Autodesk Inventor part; units mm, degrees
ref_plane "YZ Plane" through (0, 0, 0) normal (1, 0, 0) x (0, 1, 0)
ref_plane "XZ Plane" through (0, 0, 0) normal (0, 1, 0) x (-1, 0, 0)
ref_plane "XY Plane" through (0, 0, 0) normal (0, 0, 1) x (1, 0, 0)
sketch "Sketch1" plane through (0, 0, 0) normal (0, 1, 0) x (-1, 0, 0)
  line L0 (0, 25.4) -> (25.4, 25.4)
  line L1 (25.4, 25.4) -> (25.4, 0)
  line L2 (25.4, 0) -> (0, 0)
  line L3 (0, 0) -> (0, 25.4)
  line L4 (22.225, 22.225) -> (3.175, 22.225)
  line L5 (3.175, 22.225) -> (3.175, 3.175)
  line L6 (3.175, 3.175) -> (22.225, 3.175)
  line L7 (22.225, 3.175) -> (22.225, 22.225)
  dimension "d0" = 25.4
  dimension "d1" = 25.4
  dimension "d2" = 3.175
extrude "Extrusion1" add sketch "Sketch1" along normal blind 558.8
sketch "Sketch2" plane through (-25.4, 0, 25.4) normal (0, 0, 1) x (1, 0, 0)
  line L0 (25.4, 0) -> (0, 0)
  line L1 (0, 558.8) -> (25.4, 558.8)
  line L2 (12.7, 558.8) -> (12.7, 0) construction
  line L3 (12.7, 0) -> (12.7, 13.97) construction
  circle A0 centre (12.7, 13.97) radius 3.302
  circle A1 centre (12.7, 33.6315) radius 3.302
  circle A2 centre (12.7, 53.293) radius 3.302
  circle A3 centre (12.7, 72.9544) radius 3.302
  circle A4 centre (12.7, 92.6159) radius 3.302
  circle A5 centre (12.7, 112.2774) radius 3.302
  circle A6 centre (12.7, 131.9389) radius 3.302
  circle A7 centre (12.7, 151.6004) radius 3.302
  circle A8 centre (12.7, 171.2619) radius 3.302
  circle A9 centre (12.7, 190.9233) radius 3.302
  circle A10 centre (12.7, 210.5848) radius 3.302
  circle A11 centre (12.7, 230.2463) radius 3.302
  circle A12 centre (12.7, 249.9078) radius 3.302
  circle A13 centre (12.7, 269.5693) radius 3.302
  circle A14 centre (12.7, 289.2307) radius 3.302
  circle A15 centre (12.7, 308.8922) radius 3.302
  circle A16 centre (12.7, 328.5537) radius 3.302
  circle A17 centre (12.7, 348.2152) radius 3.302
  circle A18 centre (12.7, 367.8767) radius 3.302
  circle A19 centre (12.7, 387.5381) radius 3.302
  circle A20 centre (12.7, 407.1996) radius 3.302
  circle A21 centre (12.7, 426.8611) radius 3.302
  circle A22 centre (12.7, 446.5226) radius 3.302
  circle A23 centre (12.7, 466.1841) radius 3.302
  circle A24 centre (12.7, 485.8456) radius 3.302
  circle A25 centre (12.7, 505.507) radius 3.302
  circle A26 centre (12.7, 525.1685) radius 3.302
  circle A27 centre (12.7, 544.83) radius 3.302
  dimension "d5" = 13.97
  dimension "d6" = 6.604
  dimension "d7" = 558.8
  dimension "d10" = 19.6615
extrude "Extrusion2" cut sketch "Sketch2" against normal through all contours A3 | A4 | A5 | A6 | A7 | A8 | A9 | A10 | A11 | A12 | A13 | A14 | A15 | A16 | A17 | A18 | A19 | A20 | A21 | A22 | A23 | A24
sketch "Sketch3" plane through (-25.4, 0, 0) normal (-1, 0, 0) x (0, 0, 1)
  line L0 (25.4, 0) -> (25.4, 558.8)
  line L1 (0, 0) -> (0, 558.8)
  line L2 (22.225, 482.5436) -> (22.225, 489.1476) construction
  line L3 (22.225, 344.9132) -> (22.225, 351.5172) construction
  line L4 (22.225, 207.2828) -> (22.225, 213.8868) construction
  line L5 (22.225, 69.6524) -> (22.225, 76.2564) construction
  line L6 (25.4, 485.8456) -> (0, 485.8456) construction
  line L7 (0, 348.2152) -> (25.4, 348.2152) construction
  line L8 (0, 210.5848) -> (25.4, 210.5848) construction
  line L9 (0, 72.9544) -> (25.4, 72.9544) construction
  line L10 (12.7, 498.5456) -> (12.7, 454.0956) construction
  line L11 (12.7, 373.6152) -> (12.7, 322.8152) construction
  line L12 (12.7, 232.8098) -> (12.7, 188.3598) construction
  line L13 (12.7, 104.7044) -> (12.7, 60.2544) construction
  circle A0 centre (12.7, 498.5456) radius 3.302
  circle A1 centre (12.7, 454.0956) radius 3.302
  circle A2 centre (12.7, 373.6152) radius 3.302
  circle A3 centre (12.7, 322.8152) radius 3.302
  circle A4 centre (12.7, 232.8098) radius 3.302
  circle A5 centre (12.7, 188.3598) radius 3.302 construction
  circle A6 centre (12.7, 104.7044) radius 3.302
  circle A7 centre (12.7, 60.2544) radius 3.302
  line L14 (0, 279.4) -> (25.4, 279.4) construction
  line L15 (12.7, 304.8) -> (12.7, 254) construction
  circle A8 centre (12.7, 304.8) radius 3.302
  circle A9 centre (12.7, 254) radius 3.302
  line L16 (25.4, 0) -> (0, 0)
  line L17 (0, 558.8) -> (25.4, 558.8)
  circle A10 centre (12.7, 546.1) radius 3.302
  line L18 (12.7, 546.1) -> (12.7, 558.8) construction
  line L19 (12.7, 0) -> (12.7, 12.7) construction
  circle A11 centre (12.7, 12.7) radius 3.302
  line L20 (0, 82.4794) -> (25.4, 82.4794) construction
  line L21 (0, 476.3206) -> (25.4, 476.3206) construction
  line L22 (12.7, 12.7) -> (12.7, 34.8544) construction
  circle A12 centre (12.7, 34.8544) radius 3.302
  line L23 (12.7, 104.7044) -> (12.7, 130.1044) construction
  circle A13 centre (12.7, 130.1044) radius 3.302
  line L24 (12.7, 130.1044) -> (12.7, 155.5044) construction
  circle A14 centre (12.7, 155.5044) radius 3.302
  circle A15 centre (12.7, 180.9044) radius 3.302
  line L25 (12.7, 180.9044) -> (12.7, 155.5044) construction
  point P0 (22.225, 485.8456)
  point P1 (22.225, 348.2152)
  point P2 (22.225, 72.9544)
  point P3 (22.225, 210.5848)
  point P4 (12.7, 210.5848)
  point P5 (12.7, 348.2152)
  point P6 (12.7, 279.4)
  point P7 (12.7, 82.4794)
  point P8 (12.7, 476.3206)
  dimension "d17" = 44.45
  dimension "d18" = 50.8
  dimension "d19" = 44.45
  dimension "d20" = 44.45
  dimension "d21" = 6.604
  dimension "d22" = 6.604
  dimension "d23" = 6.604
  dimension "d24" = 6.604
  dimension "d25" = 6.604
  dimension "d26" = 6.604
  dimension "d27" = 6.604
  dimension "d28" = 6.604
  dimension "d31" = 50.8
  dimension "d32" = 6.604
  dimension "d33" = 6.604
  dimension "d40" = 12.7
  dimension "d41" = 6.604
  dimension "d42" = 12.7
  dimension "d43" = 6.604
  dimension "d44" = 9.525
  dimension "d45" = 9.525
  dimension "d60" = 25.4
  dimension "d61" = 6.604
  dimension "d62" = 25.4
  dimension "d63" = 6.604
  dimension "d64" = 25.4
  dimension "d65" = 6.604
extrude "Extrusion3" cut sketch "Sketch3" against normal through all contours A0 | A1 | A6 | A7 | A8 | A9 | A10 | A11 | A12 | A13 | A14 | A15
sketch "Sketch4" plane through (0, 0, 25.4) normal (1, 0, 0) x (0, 0, -1)
  circle A0 centre (12.7, 304.8) radius 3.302
  circle A1 centre (12.7, 254) radius 3.302
  line L0 (0, 0) -> (0, 558.8)
  line L1 (12.7, 304.8) -> (12.7, 323.85) construction
  line L2 (12.7, 254) -> (12.7, 234.95) construction
  circle A2 centre (12.7, 323.85) radius 3.302
  circle A3 centre (12.7, 234.95) radius 3.302
  line L3 (25.4, 0) -> (0, 0)
  line L4 (0, 558.8) -> (25.4, 558.8)
  line L5 (12.7, 558.8) -> (12.7, 0) construction
  circle A4 centre (12.7, 431.8) radius 3.302
  circle A5 centre (12.7, 406.4) radius 3.302
  circle A6 centre (12.7, 393.7) radius 3.302
  circle A7 centre (12.7, 419.1) radius 3.302
  circle A8 centre (12.7, 444.5) radius 3.302
  dimension "d46" = 19.05
  dimension "d47" = 19.05
  dimension "d48" = 6.604
  dimension "d49" = 6.604
  dimension "d52" = 6.604
  dimension "d53" = 139.7
  dimension "d54" = 12.7
  dimension "d55" = 12.7
  dimension "d56" = 12.7
  dimension "d57" = 12.7
extrude "Extrusion4" cut sketch "Sketch4" against normal blind 25.4 contours A2 | A3 | A5 | A6 | A7
equation "\"d19\" = d17"
equation "\"d20\" = d17"
equation "\"d22\" = d21"
equation "\"d23\" = d21"
equation "\"d24\" = d21"
equation "\"d25\" = d21"
equation "\"d26\" = d21"
equation "\"d27\" = d21"
equation "\"d28\" = d21"
equation "\"d31\" = d18"
equation "\"d32\" = d21"
equation "\"d33\" = d21"
equation "\"d41\" = d21"
equation "\"d42\" = d40"
equation "\"d43\" = d21"
equation "\"d45\" = d44"
equation "\"d61\" = d63"
equation "\"d55\" = d54"
equation "\"d56\" = d55"
equation "\"d57\" = d54"
properties part number "Chassis V1.500 Part4" material "Aluminum 6061"
Geometry check sheet. Reference: the model listing, model coordinates, mm. A direction names the side the tool comes from. Coordinates: 2 decimals unless noted, no trailing zeros. Order: outer loops, then holes, each group sorted by start corner. A loop starts at its lowest first (then second) coordinate and runs counter-clockwise, first axis right, second up. Notation, with made-up numbers: (-36.75, 60) - (-4.75, 60) arc R30 cw to (-4.75, 85) - close; hole circle Ø8 at (-24, 5.25). An arc over 180 degrees is marked (long way). Answer in a Markdown table with one row per item. Add a question column.
1. Gauge pin test, flat end, axial feed: pin 1 Ø12 at (x, y) = (-17, 435) entering from -Z. Record the tip position at first contact, or that the pin passes through.
2. Material ranges on L1, parallel to Z at x = -6.5, y = 31 (3 decimals); L2, parallel to X at y = 398, z = 9.75 (3 decimals); L3, parallel to Z at x = -23.1, y = 254, recorded low to high. Write a range as [from, to].
3. Access from +Z, -Z, +X, -X, +Y, -Y to the whole of each face (thin tool, end or side, straight path). Record for faces 5 (the face through (-13, 275, 22.225)), 6 (the face through (-13, 275, 0)).
4. Draft check along X on faces 1 (the face through (0, 275, 13)), 2 (the face through (-13, 275, 25.4)), 3 (the face through (-22.225, 275, 13)), 4 (the face through (-25.4, 275, 13)). Enter one of: +X half, -X half, draft (parallel to the pull), parting line (faces both ways), or undercut.
5. Section check A-A (y = 376). Enter the section's corners in (x, z) (3 decimals), plus the area to 3 significant figures.
Data:
| question | item | result |
|---|---|---|
| 1 | pin 1 | stops at z = 0 |
| 2 | L1 | z = [0, 3.175], [22.225, 25.4] |
| 2 | L2 | x = [-25.4, -22.225], [-3.175, 0] |
| 2 | L3 | z = [0, 9.4], [16, 25.4] |
| 3 | face 5 | +Y, -Y |
| 3 | face 6 | -Z, +X, -X, +Y, -Y |
| 4 | face 1 | +X half |
| 4 | face 2 | draft |
| 4 | face 3 | undercut |
| 4 | face 4 | -X half |
| 5 | outline | (-25.4, 0) - (0, 0) - (0, 25.4) - (-25.4, 25.4) - close; hole (-22.225, 3.175) - (-3.175, 3.175) - (-3.175, 22.225) - (-22.225, 22.225) - close |
| 5 | area | 282 mm² |
